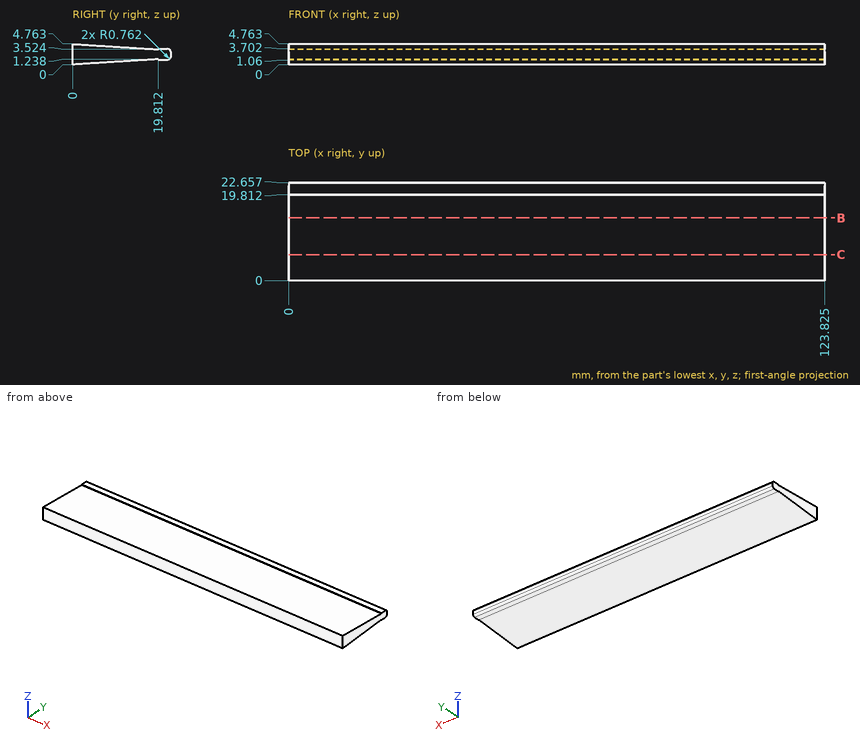
Answer from the drawing. Dimensions are ordinates in mm from the lowest x, y and z of the part. Give positions to 0.01 mm unless a question says otherwise; leave off trailing zeros. Loops run counter-clockwise (first coordinate to the right, second up) from the corner with the lowest first, then second, coordinate; pieces in that order, holes last. Notation, with made-up numbers: (41.25, -8.75) - (70.25, -8.75) arc R27 ccw to (70.25, 11.25) - close; hole circle Ø9 at (-30.5, -20.5). An arc over 180 degrees is marked (long way). Answer as CSV lines item,"result". Start each with the question number.
Item 1: Each of these flat-tipped pins is pushed along its axis until it touches: pin 1 (1 mm diameter, centred on x = 30, y = 10.5, fed in from +Z); pin 2 (4 mm diameter, centred on x = 97, y = 11, fed in from -Z); pin 3 (0.6 mm diameter, centred on x = 48.5, y = 21, fed in from -Z). Where does it stop, or does it pass through?
Item 2: A cutting plane is placed at C-C on y = 6. Determine the outline of the cut face in (x, z) (1 decimal), then the cut area to 3 significant figures.
Item 3: A cutting plane is placed at B-B on y = 14.5. Determine the outline of the cut face in (x, z) (1 decimal).
Item 4: Find the intervals of material crossed by line 1 (Y direction, x = 107.5, z = 3.05); line 2 (Z direction, x = 106.5, y = 4.5); line 3 (Z direction, x = 64.5, y = 10.75), in increasing order. Write a range as from..to.
Found:
1,pin 1,"stops at z = 4.14"
1,pin 2,"stops at z = 0.56"
1,pin 3,"stops at z = 1.06"
2,outline,"(0, 0.4) - (123.8, 0.4) - (123.8, 4.4) - (0, 4.4) - close"
2,area,"497 mm^2"
3,outline,"(0, 0.9) - (123.8, 0.9) - (123.8, 3.9) - (0, 3.9) - close"
4,line 1,"y = 0..22.65"
4,line 2,"z = 0.28..4.48"
4,line 3,"z = 0.67..4.09"
